Model file for the job. Use its own axes, mm. A direction names the side the tool comes from. Round coordinates to 2 decimals unless told otherwise and drop trailing zeros. Write each loop counter-clockwise with the first axis right and the second up, starting at its lowest first coordinate (ties: lowest second). Pieces come first, ordered by that corner, then holes.
Autodesk Inventor part; units mm, degrees
ref_plane "YZ Plane" through (0, 0, 0) normal (1, 0, 0) x (0, 1, 0)
ref_plane "XZ Plane" through (0, 0, 0) normal (0, 1, 0) x (-1, 0, 0)
ref_plane "XY Plane" through (0, 0, 0) normal (0, 0, 1) x (1, 0, 0)
sketch "Sketch1" plane through (0, 0, 0) normal (0, 0, 1) x (1, 0, 0)
  circle A0 centre (0, 0) radius 9.95
  circle A1 centre (0, 0) radius 4
  dimension "d0" = 19.9
  dimension "d1" = 8
extrude "Extrusion1" add sketch "Sketch1" along normal blind 20
sketch "Sketch2" plane through (0, 0, 20) normal (0, 0, 1) x (1, 0, 0)
  circle A0 centre (0, 0) radius 9.95
  circle A1 centre (0, 0) radius 11.95
  dimension "d4" = 23.9
extrude "Extrusion2" add sketch "Sketch2" against normal blind 4.8
chamfer "Chamfer1" distance 2 angle 45 1 edges at (-11.95, 0, 15.2)
sketch "Sketch3" plane through (0, 0, 20) normal (0, 0, 1) x (1, 0, 0)
  circle A0 centre (0, 0) radius 4
  circle A1 centre (0, 0) radius 5
  dimension "d10" = 10
extrude "Extrusion3" cut sketch "Sketch3" against normal blind 18
chamfer "Chamfer2" distance 3 distance2 13.5 1 edges at (-5, 0, 20) measured on face at (9.5176, -0.9533, 20)
properties part number "V5 Z Bottom Center Spacer"
1) Wall check: probe 1 along Y at (x, z) = (0, 0.95); probe 2 along X at (y, z) = (4, 5.75); probe 3 along X at (y, z) = (-1.5, 15.5). Give the ranges that are in metal, low to high.
2) Flat gauge pins, fed straight in: pin 1 Ø3 at (x, y) = (0, -1.5) entering from +Z; pin 2 Ø1 at (x, z) = (-7.5, 5) entering from +Y; pin 3 Ø10 at (y, z) = (-0.5, 11) entering from +X; pin 4 Ø3 at (x, y) = (4, 7.5) entering from -Z. Where does each tip first touch, or does it go through?
3) Cut at D-D on z = 18.25. List the corners of the cut face in (x, y).
4) Pull direction X, two halves, no side cores. Call faces 1 (the face through (-0.867, 3.905, 0.986)), 2 (the face through (-7.9, 6.05, 7.49)), 3 (the face through (2.855, -5.49, 11.844)), 4 (the face through (4.3, 0.1, 0)): released by +X, released by -X, zero draft, split by the parting line, or undercut.
5) Cut at C-C on z = 4.5. List the corners of the cut face in (x, y).
6) Which spindle directions (+Z, -Z, +X, -X, +Y, -Y) get a long thin tool onto all of the face, cutting with end or side? Do faces 5 (the face through (9.61, 3.026, 15.325)), 6 (the face through (-1.08, -4.88, 4.28)). Say none if no direction does.
Result sheet:
1. probe 1: y = -9.95 to -4, 4 to 9.95
1. probe 2: x = -9.11 to -3, 3 to 9.11
1. probe 3: x = -10.14 to -6.84, 6.84 to 10.14
2. pin 1: passes through
2. pin 2: stops at y = 7.07
2. pin 3: stops at x = 10.74
2. pin 4: stops at z = 0
3. outline: circle Ø23.9 at (0, 0); hole circle Ø15.22 at (0, 0)
4. face 1: undercut
4. face 2: split by the parting line
4. face 3: undercut
4. face 4: zero draft
5. outline: circle Ø19.9 at (0, 0); hole circle Ø10 at (0, 0)
6. face 5: -Z
6. face 6: +Z
